Geometry check sheet. Reference: drawing and pictorial views, mm from the part's lowest x, y, z. A direction names the side the tool comes from. Coordinates: 2 decimals unless noted, no trailing zeros. Order: outer loops, then holes, each group sorted by start corner. A loop starts at its lowest first (then second) coordinate and runs counter-clockwise, first axis right, second up. Notation, with made-up numbers: M -33.5,-31 L 25.5,-31 A11 ccw 25.5,-21 Z; hole C -30.5,4 d11. An arc over 180 degrees is marked long. Return JSON: item names as keys, results as strings.
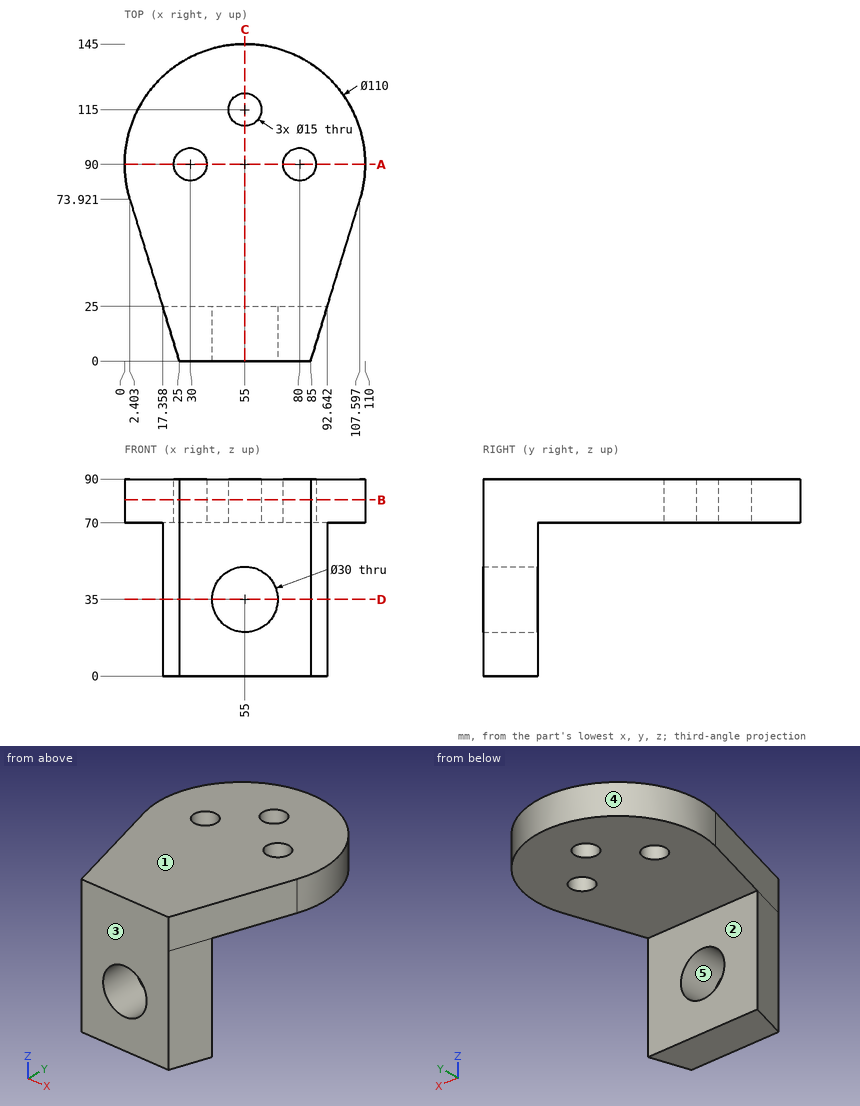
Q1. Cross-section at A-A, the plane y = 90. Record the boundary of the cut face in (x, z), and give its area (3 significant figures).
Values:
{"outline": "M 0,70 L 22.5,70 L 22.5,90 L 0,90 Z; M 37.5,70 L 72.5,70 L 72.5,90 L 37.5,90 Z; M 87.5,70 L 110,70 L 110,90 L 87.5,90 Z", "area": "1,600 mm^2"}
Q2. Cross-section at C-C, the plane x = 55. Record the boundary of the cut face in (y, z).
Values:
{"outline": "M 0,0 L 25,0 L 25,20 L 0,20 Z; M 0,50 L 25,50 L 25,70 L 107.5,70 L 107.5,90 L 0,90 Z; M 122.5,70 L 145,70 L 145,90 L 122.5,90 Z"}
Q3. Draft check along Y on the marked faces 3, 4 and 5. Enter one of: pulls with the +Y half, pulls with the -Y half, needs draft (parallel to the pull), parting line crosses it, or undercut.
Values:
{"face 3": "pulls with the -Y half", "face 4": "parting line crosses it", "face 5": "needs draft"}
Q4. Cross-section at D-D, the plane z = 35. Record the boundary of the cut face in (x, y).
Values:
{"outline": "M 17.36,25 L 25,0 L 40,0 L 40,25 Z; M 70,0 L 85,0 L 92.64,25 L 70,25 Z"}
Q5. Tool access check on the marked faces 1 and 2. Record the directions out of +Z, -Z, +X, -X, +Y, -Y that give a thin tool (end or side, any length) a straight path to the whole face; none if there is none.
Values:
{"face 1": "+Z, +X, -X, +Y, -Y", "face 2": "-Z, +X, -X, +Y"}
Q6. Material ranges on line 1 along Y through (x, z) = (55, 79.5); line 2 along Z through (x, y) = (55, 9); line 3 along Z through (x, y) = (88, 117), recorded low to high.
Values:
{"line 1": "0 to 107.5, 122.5 to 145", "line 2": "0 to 20, 50 to 90", "line 3": "70 to 90"}
Q7. Go/stop test with flat-tipped pins: pin 1 (5 mm diameter, centred on x = 72, z = 46.5, fed in from +Y); pin 2 (2 mm diameter, centred on x = 59.5, y = 105, fed in from -Z). Record where each tip stops, or that it passes through.
Values:
{"pin 1": "y = 25", "pin 2": "z = 70"}
Q8. Cross-section at B-B, the plane z = 80.5. Record the boundary of the cut face in (x, y).
Values:
{"outline": "M 2.4,73.92 L 25,0 L 85,0 L 107.6,73.92 A55 ccw long Z; hole C 30,90 d15; hole C 55,115 d15; hole C 80,90 d15"}
